For this review, use the dimensioned drawing (mm, ordinates from the lowest corner) and the shaded views. A direction names the side the tool comes from. Coordinates: 2 decimals unless noted, no trailing zeros. Order: outer loops, then holes, each group sorted by start corner. A loop starts at its lowest first (then second) coordinate and runs counter-clockwise, first axis right, second up. Notation, with made-up numbers: M 61.25,77 L 106.25,77 A9 cw 106.25,91 Z; hole C 65,67.25 d7. An arc over 180 degrees is marked long. Answer in a Markdown table with one row per item.
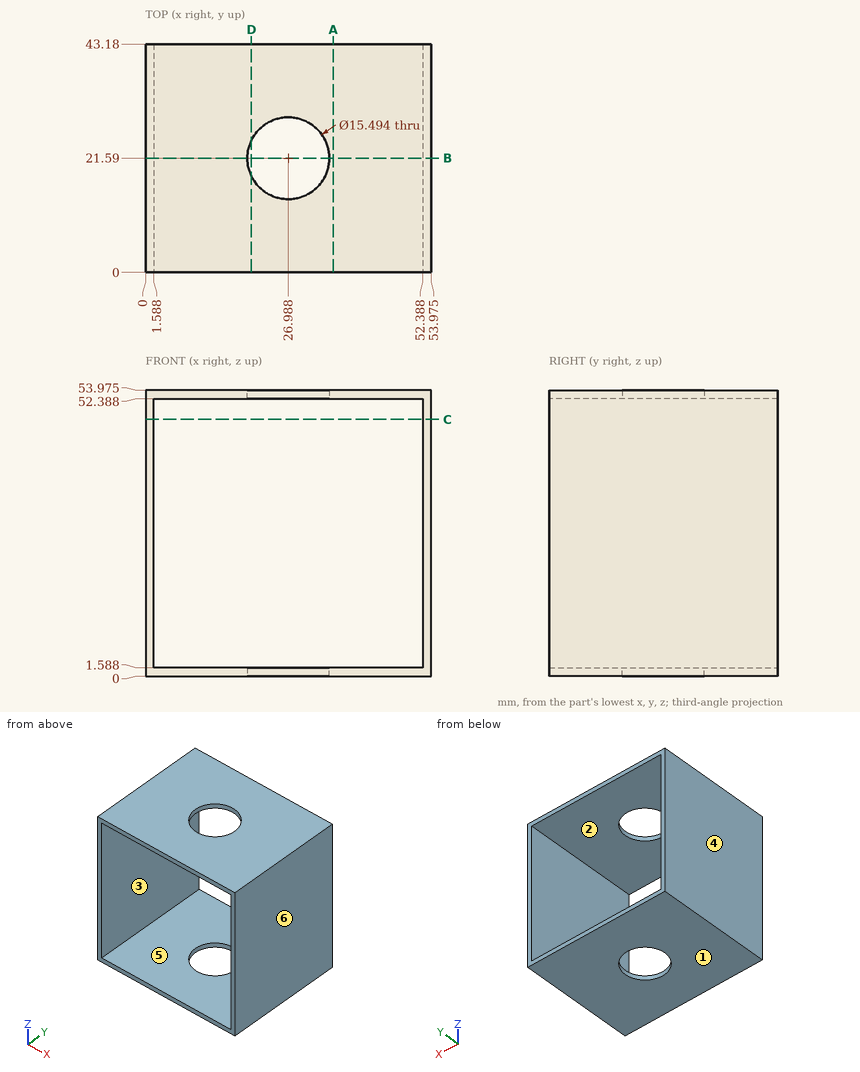
(1) Add section D-D, the plane x = 20. Give the boundary of the cut face in (y, z) (1 decimal).
Return value:
| item | result |
|---|---|
| outline | M 0,0 L 18.2,0 L 18.2,1.6 L 0,1.6 Z; M 0,52.4 L 18.2,52.4 L 18.2,54 L 0,54 Z; M 24.9,0 L 43.2,0 L 43.2,1.6 L 24.9,1.6 Z; M 24.9,52.4 L 43.2,52.4 L 43.2,54 L 24.9,54 Z |
(2) Add section A-A, the plane x = 35.5. Give the boundary of the cut face in (y, z) (1 decimal).
Return value:
| item | result |
|---|---|
| outline | M 0,0 L 43.2,0 L 43.2,1.6 L 0,1.6 Z; M 0,52.4 L 43.2,52.4 L 43.2,54 L 0,54 Z |
(3) Add section C-C, the plane z = 48.5. Give the boundary of the cut face in (x, y) (1 decimal), and give its area (3 significant figures).
Return value:
| item | result |
|---|---|
| outline | M 0,0 L 1.6,0 L 1.6,43.2 L 0,43.2 Z; M 52.4,0 L 54,0 L 54,43.2 L 52.4,43.2 Z |
| area | 137 mm2 |
(4) Insertion check: pin 1 Ø13 at (x, y) = (23.5, 23) entering from +Z (1 decimal). The pin has a flat end and moves straight along its axis. Give the tip position at first contact, or say it passes through.
Return value:
| item | result |
|---|---|
| pin 1 | stops at z = 54 |
(5) Draft analysis for pull direction X (two halves, no side actions). For the marked faces 3, 4, 5 and 6, state which applies: pulls with the +X half, pulls with the -X half, needs draft (parallel to the pull), parting line crosses it, or undercut.
Return value:
| item | result |
|---|---|
| face 3 | undercut |
| face 4 | pulls with the -X half |
| face 5 | undercut |
| face 6 | pulls with the +X half |
(6) For line 1 along X through (y, z) = (39.5, 18) (1 decimal), list the stretches that pass through material, from the lowest coordinate up. Write a range as from..to.
Return value:
| item | result |
|---|---|
| line 1 | x = 0..1.6, 52.4..54 |
(7) For the marked faces 1 and 2, list the 3-axis set-ups (+Z, -Z, +X, -X, +Y, -Y) from which the entire face can be reached by the end or side of a thin tool; tool diameter is ignored.
Return value:
| item | result |
|---|---|
| face 1 | -Z, +X, -X, +Y, -Y |
| face 2 | +Y, -Y |
(8) Add section B-B, the plane y = 21.59. Give the boundary of the cut face in (x, z) (1 decimal).
Return value:
| item | result |
|---|---|
| outline | M 0,0 L 19.2,0 L 19.2,1.6 L 1.6,1.6 L 1.6,52.4 L 19.2,52.4 L 19.2,54 L 0,54 Z; M 34.7,0 L 54,0 L 54,54 L 34.7,54 L 34.7,52.4 L 52.4,52.4 L 52.4,1.6 L 34.7,1.6 Z |
